Answer from the drawing. Dimensions are ordinates in mm from the lowest x, y and z of the part. A direction names the side the tool comes from. Coordinates: 2 decimals unless noted, no trailing zeros. Write each loop counter-clockwise with the first axis right and the second up, starting at its lowest first coordinate (ties: lowest second). Pieces come first, ordered by that corner, then holes. Notation, with made-up numbers: (-29.5, 75.25) - (5.5, 75.25) arc R37 ccw to (5.5, 114.25) - close; hole circle Ø11 at (-39, -32.75). An arc over 180 degrees is marked (long way). Answer as a JSON object with one key per item and string values. Group by question number.
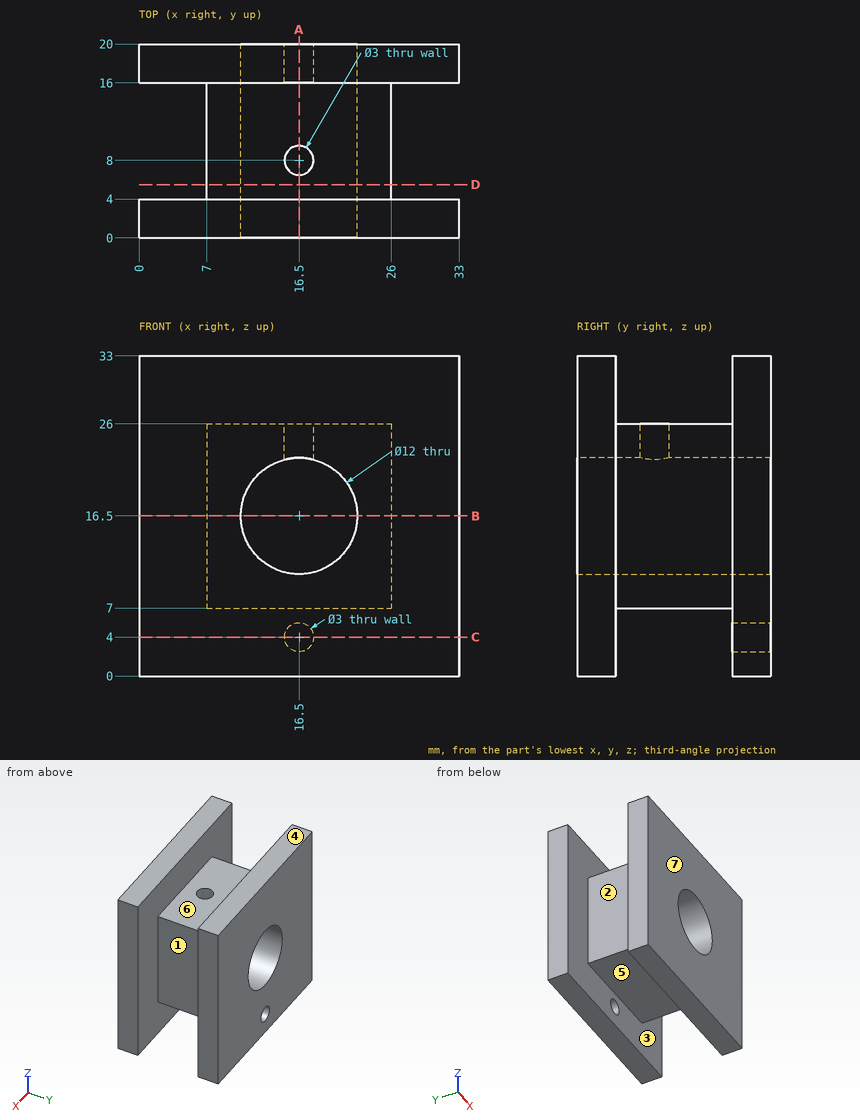
Q1. Consider L1, parallel to Y at x = 20.5, z = 2.5; L2, parallel to X at y = 8, z = 23.8; L3, parallel to X at y = 8.75, z = 16.5. Determine where each line is inside the solid, lowest interval first. Write a range as from..to.
Q2. A tool of negligible diameter and unlimited length cuts with its end or side. For the marked faces 1, 2 and 3, from which of +Z, -Z, +X, -X, +Y, -Y can it reach the whole face along a straight path? Write none if from no direction.
Q3. Flat-ended cylindrical pins translate along their axes: pin 1 Ø11 at (x, z) = (16.5, 16.5) entering from -Y; pin 2 Ø6 at (x, y) = (21, 12.5) entering from -Z; pin 3 Ø5 at (y, z) = (12, 21.5) entering from -X; pin 4 Ø2.5 at (x, z) = (16.5, 4) entering from +Y. Find the tip coordinate at first contact, or state that the pin passes through.
Q4. Section B-B on z = 16.5 is taken. Determine the outline of the cut face in (x, y), plus the area to 3 significant figures.
Q5. Section A-A on x = 16.5 is taken. Determine the outline of the cut face in (y, z), plus the area to 4 significant figures.
Q6. For a pull along Y with two mould halves and no side action, classify the marked faces 4, 5, 6 and 7 as +Y half, -Y half, draft (parallel to the pull), parting line (faces both ways), or undercut.
Q7. Section D-D on y = 5.5 is taken. Determine the outline of the cut face in (x, z).
Q8. Section C-C on z = 4 is taken. Determine the outline of the cut face in (x, y).
Numbers:
{
 "1": {"L1": "y = 0..4, 16..20", "L2": "x = 7..15, 18..26", "L3": "x = 7..10.5, 22.5..26"},
 "2": {"face 1": "+Z, -Z, +X", "face 2": "+Z, -Z, -X", "face 3": "none"},
 "3": {"pin 1": "passes through", "pin 2": "stops at z = 7", "pin 3": "stops at x = 7", "pin 4": "stops at y = 4"},
 "4": {"outline": "(0, 0) - (10.5, 0) - (10.5, 20) - (0, 20) - (0, 16) - (7, 16) - (7, 4) - (0, 4) - close; (22.5, 0) - (33, 0) - (33, 4) - (26, 4) - (26, 16) - (33, 16) - (33, 20) - (22.5, 20) - close", "area": "252 mm²"},
 "5": {"outline": "(0, 0) - (4, 0) - (4, 7) - (16, 7) - (16, 5.5) - (20, 5.5) - (20, 10.5) - (0, 10.5) - close; (0, 22.5) - (6.5, 22.5) - (6.5, 26) - (4, 26) - (4, 33) - (0, 33) - close; (9.5, 22.5) - (20, 22.5) - (20, 33) - (16, 33) - (16, 26) - (9.5, 26) - close; (16, 0) - (20, 0) - (20, 2.5) - (16, 2.5) - close", "area": "229.5 mm²"},
 "6": {"face 4": "draft", "face 5": "undercut", "face 6": "undercut", "face 7": "-Y half"},
 "7": {"outline": "(7, 7) - (26, 7) - (26, 26) - (7, 26) - close; hole circle Ø12 at (16.5, 16.5)"},
 "8": {"outline": "(0, 0) - (33, 0) - (33, 4) - (0, 4) - close; (0, 16) - (15, 16) - (15, 20) - (0, 20) - close; (18, 16) - (33, 16) - (33, 20) - (18, 20) - close"}
}
